```python
from build123d import *

# Parameters (mm, degrees)
SKETCH1_W               = 70
SKETCH1_H               = 80
BOSS_EXTRUDE1_DEPTH     = 55
CUT_EXTRUDE1_DEPTH      = 104.198837203
CUT_EXTRUDE1_DEPTH_BACK = 104.198837203
SKETCH2_W               = 27.5
SKETCH2_H               = 30
SHELL1_T                = -3
CUT_EXTRUDE2_DEPTH      = 101.891030325
SKETCH9_R               = 2
CUT_EXTRUDE3_DEPTH      = 102.631687972
LPATTERN1_COUNT         = 2
LPATTERN1_PITCH         = 40
LPATTERN1_COUNT_DIR2    = 2
LPATTERN1_PITCH_DIR2    = 50


with BuildPart() as part:
    # Sketch1 → Boss-Extrude1 (new body)
    with BuildSketch(Plane.XY):
        with Locations((0, -40)):
            Rectangle(SKETCH1_W, SKETCH1_H)
    extrude(amount=BOSS_EXTRUDE1_DEPTH)

    # Sketch2 → Cut-Extrude1 (cut, two sides: drawn at the far end of the back side and taken through both)
    with BuildSketch(Plane(origin=(0, 0, 0), x_dir=(0, 0, -1), z_dir=(1, 0, 0)).offset(-CUT_EXTRUDE1_DEPTH_BACK)):
        with Locations((-41.25, -15)):
            Rectangle(SKETCH2_W, SKETCH2_H)
    extrude(amount=CUT_EXTRUDE1_DEPTH + CUT_EXTRUDE1_DEPTH_BACK, mode=Mode.SUBTRACT)

    # Shell1
    shell1_openings = [part.faces().sort_by_distance(p)[0] for p in [
        (0, 0, 13.75),
        (35, -45.769230769, 24.326923077),
        (0, -15, 27.5),
        (-35, -45.769230769, 24.326923077),
        (0, -30, 41.25),
    ]]
    offset(amount=SHELL1_T, openings=shell1_openings, kind=Kind.INTERSECTION)

    # Sketch8 → Cut-Extrude2 (cut, through all)
    with BuildSketch(Plane(origin=(0, -77, 0), x_dir=(1, 0, 0), z_dir=(0, 1, 0))):
        with BuildLine():
            Line((-26.5, -23.45), (-35, -23.45))
            Line((-35, -23.45), (-35, -31.55))
            Line((-35, -31.55), (-26.5, -31.55))
            ThreePointArc((-26.5, -31.55), (-22.45, -27.5), (-26.5, -23.45))
        make_face()
    extrude(amount=-CUT_EXTRUDE2_DEPTH, mode=Mode.SUBTRACT)

    # Sketch9 → Cut-Extrude3 (cut, through all)
    with BuildSketch(Plane.XY.offset(3)):
        with Locations((-30, -5)):
            Circle(SKETCH9_R)
        with Locations((-10, -5)):
            Circle(SKETCH9_R)
        with Locations((-30, -23)):
            Circle(SKETCH9_R)
        with Locations((-10, -23)):
            Circle(SKETCH9_R)
    cut_extrude3 = extrude(amount=-CUT_EXTRUDE3_DEPTH, mode=Mode.SUBTRACT)

    # LPattern1: Cut-Extrude3 2 × 2
    with Locations(*[(i * LPATTERN1_PITCH, -j * LPATTERN1_PITCH_DIR2, 0) for i in range(LPATTERN1_COUNT) for j in range(LPATTERN1_COUNT_DIR2) if (i, j) != (0, 0)]):
        add(cut_extrude3, mode=Mode.SUBTRACT)


solid = part.part
```
The model under review builds one solid part; all positions refer to its coordinate system, in mm. A direction names the side the tool comes from. Round coordinates to 2 decimals unless told otherwise and drop trailing zeros. Order: outer loops, then holes, each group sorted by start corner. A loop starts at its lowest first (then second) coordinate and runs counter-clockwise, first axis right, second up.
(1) For P1, Ø10, axis at x = -10, z = 35, coming from the +Y side; P2, Ø3, axis at x = 30, y = -73, coming from the -Z side; P3, Ø3.5, axis at x = -10, y = -5, coming from the -Z side; P4, Ø5, axis at x = -30, y = -23, coming from the +Z side, all flat-tipped, find the tip position at first contact; note any pin that passes through.
Working result:
P1: stops at y = -77
P2: stops at z = 52
P3: passes through
P4: stops at z = 3
(2) Take a section at D-D, the plane x = 7. State the section outline as (y, z) points, plus the area to 3 significant figures.
Working result:
outline: (-80, 0) - (0, 0) - (0, 3) - (-77, 3) - (-77, 52) - (-30, 52) - (-30, 55) - (-80, 55) - close
area: 537 mm2
(3) Wall thickness on L1, parallel to Y at x = -30, z = 1; L2, parallel to Z at x = 16.5, y = -57; L3, parallel to Y at x = 27, z = 47: over which ranges is each line inside the solid? List them lowest first.
Working result:
L1: y = -80 to -75, -71 to -57, -53 to -25, -21 to -7, -3 to 0
L2: z = 0 to 3, 52 to 55
L3: y = -80 to -77
(4) Take a section at C-C, the plane y = -23. State the section outline as (x, z) points.
Working result:
outline: (-35, 0) - (-32, 0) - (-32, 3) - (-35, 3) - close; (-28, 0) - (-12, 0) - (-12, 3) - (-28, 3) - close; (-8, 0) - (8, 0) - (8, 3) - (-8, 3) - close; (12, 0) - (28, 0) - (28, 3) - (12, 3) - close; (32, 0) - (35, 0) - (35, 3) - (32, 3) - close
(5) Tool access review of faces 1 (the face through (-31, -78, 23.45)), 2 (the face through (-28.092, -54.399, 1.521)), 3 (the face through (0, -38, 3)): name each direction out of +Z, -Z, +X, -X, +Y, -Y from which nothing blocks a thin tool from reaching the whole face with its end or side.
Working result:
face 1: -X, +Y, -Y
face 2: -Z
face 3: +X, -X, +Y
(6) Take a section at B-B, the plane y = -73. State the section outline as (x, z) points.
Working result:
outline: (-35, 0) - (-32, 0) - (-32, 3) - (-35, 3) - close; (-35, 52) - (35, 52) - (35, 55) - (-35, 55) - close; (-28, 0) - (-12, 0) - (-12, 3) - (-28, 3) - close; (-8, 0) - (8, 0) - (8, 3) - (-8, 3) - close; (12, 0) - (28, 0) - (28, 3) - (12, 3) - close; (32, 0) - (35, 0) - (35, 3) - (32, 3) - close
(7) Mouldability with a two-part tool opening along Y and no side actions: class faces 4 (the face through (0, -30, 54)), 5 (the face through (-10, -53, 2)), 6 (the face through (-35, -64, 53)) as released by +Y, released by -Y, zero draft, split by the parting line, or undercut.
Working result:
face 4: released by +Y
face 5: undercut
face 6: zero draft
(8) Take a section at A-A, the plane x = -10. State the section outline as (y, z) points.
Working result:
outline: (-80, 0) - (-75, 0) - (-75, 3) - (-77, 3) - (-77, 52) - (-30, 52) - (-30, 55) - (-80, 55) - close; (-71, 0) - (-57, 0) - (-57, 3) - (-71, 3) - close; (-53, 0) - (-25, 0) - (-25, 3) - (-53, 3) - close; (-21, 0) - (-7, 0) - (-7, 3) - (-21, 3) - close; (-3, 0) - (0, 0) - (0, 3) - (-3, 3) - close
